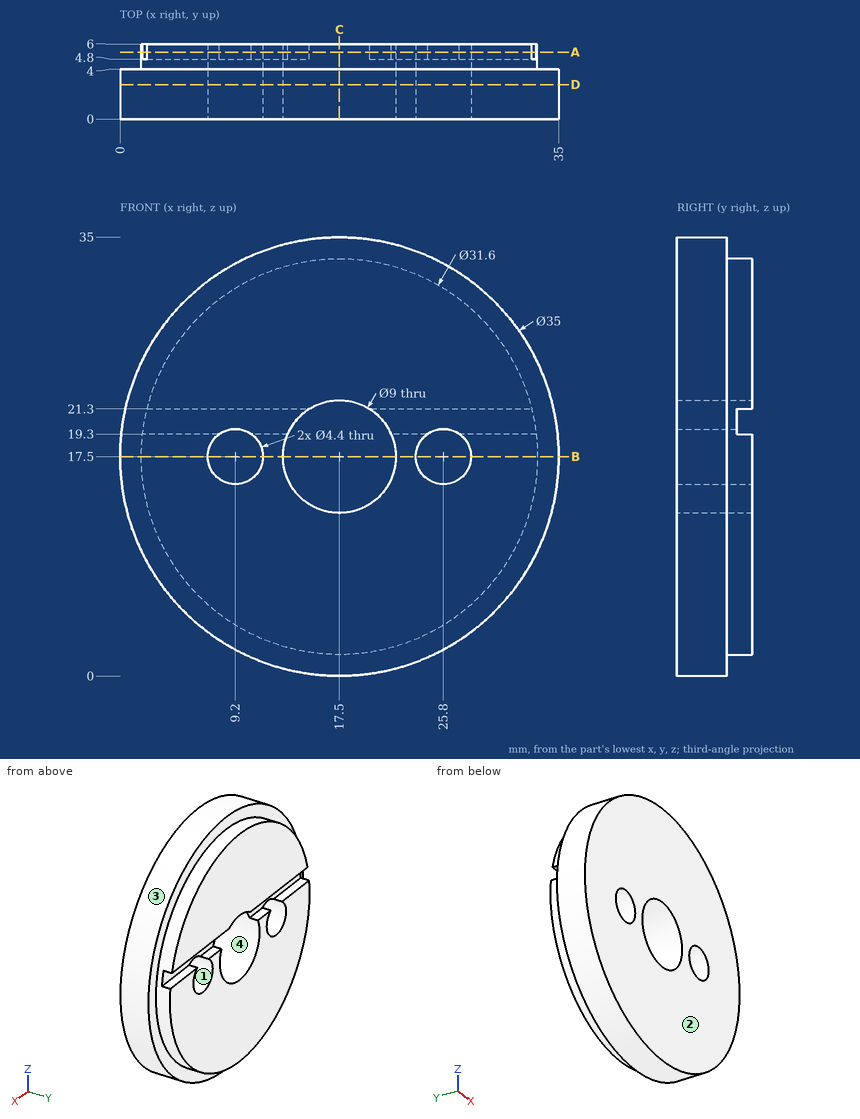
Geometry check sheet. Reference: drawing and pictorial views, mm from the part's lowest x, y, z. Round coordinates to 2 decimals unless told otherwise and drop trailing zeros. Order: outer loops, then holes, each group sorted by start corner. A loop starts at its lowest first (then second) coordinate and runs counter-clockwise, first axis right, second up. Notation, with made-up numbers: (69.5, 76.5) - (77.5, 76.5) arc R19 cw to (77.5, 92.5) - close; hole circle Ø6 at (6.5, 66). An arc over 180 degrees is marked (long way). Use a Markdown table: item, result. Add a question column.
1) Gauge pin test, flat ends, axial feed: P1, Ø7, axis at x = 17.5, z = 17.5, coming from the +Y side; P2, Ø12, axis at x = 11, z = 8, coming from the -Y side; P3, Ø1.3, axis at x = 22.5, y = 5.5, coming from the +Z side; P4, Ø1, axis at x = 12, y = 5.5, coming from the +Z side. Record the tip position at first contact, or that the pin passes through.
2) Thickness scan on line 1 along X through (y, z) = (3.6, 17.5); line 2 along Z through (x, y) = (14.5, 4.5); line 3 along Z through (x, y) = (19.5, 0.8). Record the ranges inside material, lowest first.
3) Section check D-D (y = 2.75). Record the cut outline in (x, z), then the cut area to 3 significant figures.
4) Section check B-B (z = 17.5). Record the cut outline in (x, y).
5) Section check A-A (y = 5.35). Record the cut outline in (x, z).
6) Mould release check, pull along Z, two halves, no side actions. Record for the marked faces 1, 2, 3 and 4: released by +Z, released by -Z, zero draft, split by the parting line, or undercut.
7) Section check C-C (x = 17.5). Record the cut outline in (y, z), then the cut area to 3 significant figures.
Established:
| question | item | result |
|---|---|---|
| 1 | P1 | through |
| 1 | P2 | y = 0 |
| 1 | P3 | z = 32.69 |
| 1 | P4 | z = 32.49 |
| 2 | line 1 | 0 to 7, 11.4 to 13, 22 to 23.6, 28 to 35 |
| 2 | line 2 | 1.99 to 14.15, 20.85 to 33.01 |
| 2 | line 3 | 0.11 to 13.47, 21.53 to 34.89 |
| 3 | outline | circle Ø35 at (17.5, 17.5); hole circle Ø4.4 at (9.2, 17.5); hole circle Ø9 at (17.5, 17.5); hole circle Ø4.4 at (25.8, 17.5) |
| 3 | area | 868 mm2 |
| 4 | outline | (0, 0) - (7, 0) - (7, 6) - (1.7, 6) - (1.7, 4) - (0, 4) - close; (11.4, 0) - (13, 0) - (13, 6) - (11.4, 6) - close; (22, 0) - (23.6, 0) - (23.6, 6) - (22, 6) - close; (28, 0) - (35, 0) - (35, 4) - (33.3, 4) - (33.3, 6) - (28, 6) - close |
| 5 | outline | (1.8, 19.3) arc R15.8 ccw (long way) to (33.2, 19.3) - (27.06, 19.3) arc R2.2 cw (long way) to (24.54, 19.3) - (21.62, 19.3) arc R4.5 cw (long way) to (13.38, 19.3) - (10.46, 19.3) arc R2.2 cw (long way) to (7.94, 19.3) - close; (2.16, 21.3) - (15.09, 21.3) arc R4.5 cw to (19.91, 21.3) - (32.84, 21.3) arc R15.8 ccw to start |
| 6 | face 1 | undercut |
| 6 | face 2 | zero draft |
| 6 | face 3 | split by the parting line |
| 6 | face 4 | undercut |
| 7 | outline | (0, 0) - (4, 0) - (4, 1.7) - (6, 1.7) - (6, 13) - (0, 13) - close; (0, 22) - (6, 22) - (6, 33.3) - (4, 33.3) - (4, 35) - (0, 35) - close |
| 7 | area | 149 mm2 |
